The drawing under review shows one solid part. Ordinate dimensions are in mm from its lowest x, y, z. A direction names the side the tool comes from. Round coordinates to 2 decimals unless told otherwise and drop trailing zeros. Order: outer loops, then holes, each group sorted by start corner. A loop starts at its lowest first (then second) coordinate and runs counter-clockwise, first axis right, second up. Notation, with made-up numbers: (33, -16.75) - (38, -16.75) arc R10 cw to (38, -7.75) - close; hole circle Ø11 at (61.5, 38). An arc over 180 degrees is marked (long way). One line per question, with ' | ' between items.
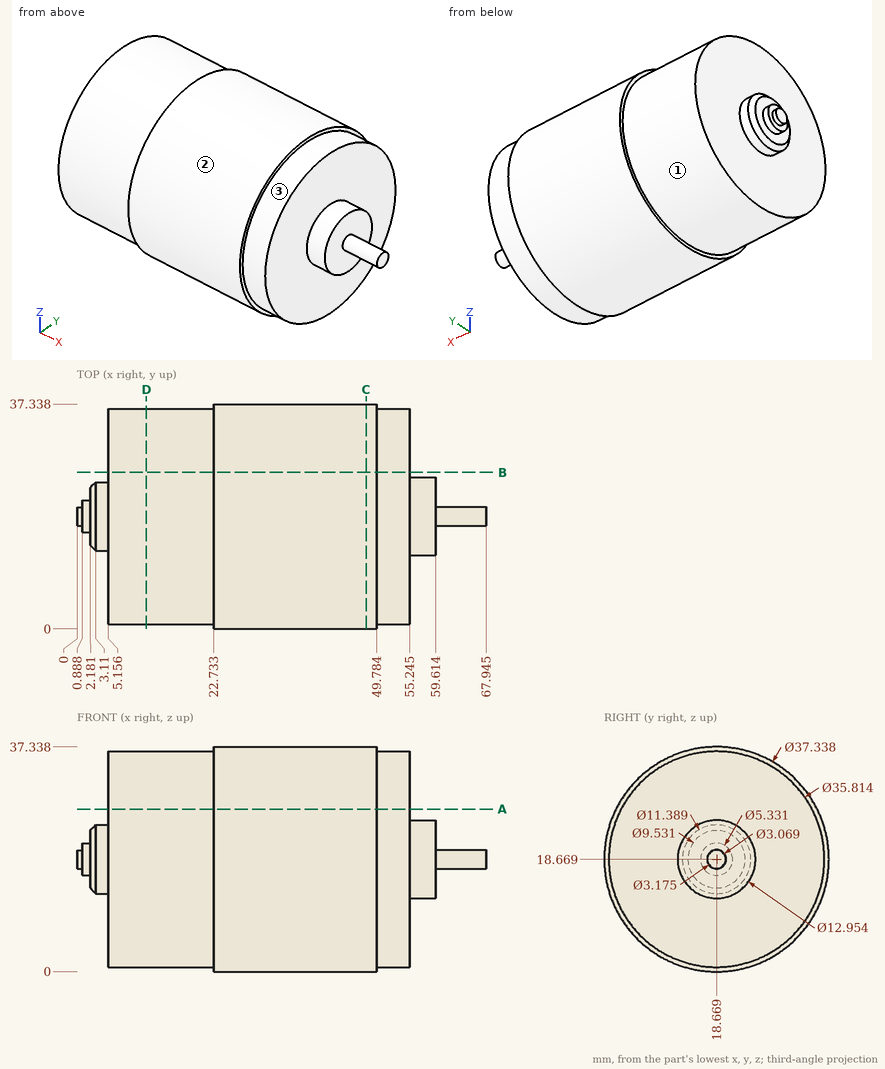
(1) For probe 1 along X at (y, z) = (22, 3) (1 decimal); probe 2 along Y at (x, z) = (31.5, 20.5); probe 3 along Y at (x, z) = (40, 13) (1 decimal), list the stretches that pass through material, from the lowest coordinate up. Write a range as [from, to].
Output values:
probe 1: [5.2, 55.2] | probe 2: [0.09, 37.25] | probe 3: [0.9, 36.5]
(2) We need section D-D on x = 11.5. State the section outline as (y, z) points, plus the area to 3 significant figures.
Output values:
outline: circle Ø35.81 at (18.67, 18.67) | area: 1,010 mm^2
(3) For the marked faces 1, 2 and 3, list the 3-axis set-ups (+Z, -Z, +X, -X, +Y, -Y) from which the entire face can be reached by the end or side of a thin tool; tool diameter is ignored.
Output values:
face 1: -X | face 2: +X, -X | face 3: +X
(4) Insertion check: pin 1 (5 mm diameter, centred on x = 14, z = 8, fed in from -Y) (1 decimal); pin 2 (10 mm diameter, centred on y = 17, z = 27.5, fed in from -X); pin 3 (6 mm diameter, centred on y = 10.5, z = 4, fed in from +X) (3 decimals); pin 4 (10.5 mm diameter, centred on y = 18.5, z = 14, fed in from -X). Each pin has a flat end and moves straight along its axis. Give the tip position at first contact, or say it passes through.
Output values:
pin 1: y = 2.7 | pin 2: x = 2.18 | pin 3: x = 55.245 | pin 4: x = 0
(5) We need section B-B on y = 26. State the section outline as (x, z) points (1 decimal), plus the area to 3 significant figures.
Output values:
outline: (5.2, 2.3) - (22.7, 2.3) - (22.7, 1.5) - (49.8, 1.5) - (49.8, 2.3) - (55.2, 2.3) - (55.2, 35) - (49.8, 35) - (49.8, 35.8) - (22.7, 35.8) - (22.7, 35) - (5.2, 35) - close | area: 1,680 mm^2
(6) We need section A-A on z = 27. State the section outline as (x, y) points (1 decimal), plus the area to 3 significant figures.
Output values:
outline: (5.2, 2.8) - (22.7, 2.8) - (22.7, 2) - (49.8, 2) - (49.8, 2.8) - (55.2, 2.8) - (55.2, 34.5) - (49.8, 34.5) - (49.8, 35.4) - (22.7, 35.4) - (22.7, 34.5) - (5.2, 34.5) - close | area: 1,630 mm^2
(7) We need section C-C on x = 48. State the section outline as (y, z) points, plus the area to 4 significant figures.
Output values:
outline: circle Ø37.34 at (18.67, 18.67) | area: 1,095 mm^2
